Can you work these out from the model? Positions are in its coordinate system, mm. A direction names the side the tool comes from. Round coordinates to 2 decimals unless told otherwise and drop trailing zeros. Order: outer loops, then holes, each group sorted by start corner. A loop starts at its lowest first (then second) coordinate and runs counter-clockwise, first axis right, second up. Notation, with made-up numbers: (61, 36) - (109, 36) arc R27 cw to (109, 64) - close; hole circle Ø1 at (18.25, -26). An arc over 180 degrees is marked (long way). Write item = value, one per line.
from build123d import *

# Parameters (mm, degrees)
F0_R          = 40
F0_R_2        = 2
F0_R_3        = 30
F1_DEPTH      = 8
F2_R          = 40
F2_R_2        = 30
F3_DEPTH      = 2
F4_R          = 5
F5_DEPTH      = 30
F5_DEPTH_BACK = 30
F6_W          = 8
F6_H          = 1


with BuildPart() as f1:
    # F0 (on Top) → F1 (new body)
    with BuildSketch(Plane.XY):
        Circle(F0_R)
        with Locations((-30.310889, -17.5)):
            Circle(F0_R_2, mode=Mode.SUBTRACT)
        with Locations((0, -35)):
            Circle(F0_R_2, mode=Mode.SUBTRACT)
        with Locations((30.310889, -17.5)):
            Circle(F0_R_2, mode=Mode.SUBTRACT)
        with Locations((-30.310889, 17.5)):
            Circle(F0_R_2, mode=Mode.SUBTRACT)
        Circle(F0_R_3, mode=Mode.SUBTRACT)
        with Locations((30.310889, 17.5)):
            Circle(F0_R_2, mode=Mode.SUBTRACT)
        with Locations((0, 35)):
            Circle(F0_R_2, mode=Mode.SUBTRACT)
    extrude(amount=F1_DEPTH)

    # F2 (on face) → F3 (join)
    with BuildSketch(Plane.XY.offset(8)):
        Circle(F2_R)
        Circle(F2_R_2, mode=Mode.SUBTRACT)
    extrude(amount=F3_DEPTH)

    # F4 (on Front) → F5 (join, two sides)
    with BuildSketch(Plane.XZ) as f5_sk:
        with Locations((0, 5)):
            Circle(F4_R)
    extrude(amount=F5_DEPTH)
    extrude(f5_sk.sketch, amount=-F5_DEPTH_BACK)

    # F6 (on Right) → F7 (revolve, cut)
    with BuildSketch(Plane.YZ):
        with Locations((11, 9.5)):
            Rectangle(F6_W, F6_H)
        with Locations((-11, 9.5)):
            Rectangle(F6_W, F6_H)
    revolve(axis=Axis((0, 0, 5), (0, -1, 0)), mode=Mode.SUBTRACT)


solid = f1.part
(1) Will these pins go through, and if not, where does the flat tip stop? P1, Ø2, axis at y = -12.5, z = 2, coming from the -X side; P2, Ø1.5, axis at y = -13, z = 7, coming from the -X side; P3, Ø1.2, axis at x = 30, y = 17.5, coming from the -Z side.
Computed:
P1 = -38.31
P2 = -38.08
P3 = 8
(2) If I drill on line 1 (Y direction, x = 0, z = 3.5); line 2 (Y direction, x = -2, z = 9.5); line 3 (Y direction, x = 17.5, z = 2.5), over which ranges is the centre line in solid material (lowest first)? Write a range as from..to.
Computed:
line_1 = -40..-37, -33..33, 37..40
line_2 = -39.95..-15, -7..7, 15..39.95
line_3 = -35.97..-24.37, 24.37..35.97
(3) If we section it at D-D (x = -3): Write out the boundary of the cut face in (y, z), plus the area to 3 significant figures.
Computed:
outline = (-39.89, 0) - (-29.85, 0) - (-29.85, 1) - (-15, 1) - (-15, 2.35) - (-7, 2.35) - (-7, 1) - (7, 1) - (7, 2.35) - (15, 2.35) - (15, 1) - (29.85, 1) - (29.85, 0) - (39.89, 0) - (39.89, 10) - (29.85, 10) - (29.85, 9) - (15, 9) - (15, 7.65) - (7, 7.65) - (7, 9) - (-7, 9) - (-7, 7.65) - (-15, 7.65) - (-15, 9) - (-29.85, 9) - (-29.85, 10) - (-39.89, 10) - close
area = 635 mm^2
(4) If we section it at B-B (x = 15): Write out the boundary of the cut face in (y, z).
Computed:
outline = (-37.08, 0) - (-25.98, 0) - (-25.98, 10) - (-37.08, 10) - close; (25.98, 0) - (37.08, 0) - (37.08, 10) - (25.98, 10) - close
(5) If we section it at C-C (y = 22): Write out the boundary of the cut face in (x, z), plus the area to 3 significant figures.
Computed:
outline = (-33.41, 0) - (-20.4, 0) - (-20.4, 10) - (-33.41, 10) - close; circle Ø10 at (0, 5); (20.4, 0) - (33.41, 0) - (33.41, 10) - (20.4, 10) - close
area = 339 mm^2
(6) If we section it at A-A (y = 0): Write out the boundary of the cut face in (x, z).
Computed:
outline = (-40, 0) - (-30, 0) - (-30, 10) - (-40, 10) - close; circle Ø10 at (0, 5); (30, 0) - (40, 0) - (40, 10) - (30, 10) - close
(7) Thinking about a two-plate mould opening in Y: for faces 1 (the face through (-6, 30, 0)), 2 (the face through (29.993, -0.66, 4.93)), 3 (the face through (-8.67, -39.05, 4.93)), which applies, +Y half, -Y half, draft (parallel to the pull), parting line (faces both ways), or undercut?
Computed:
face_1 = draft
face_2 = undercut
face_3 = parting line
(8) On a 3-axis mill with a long thin cutter (end or side, diameter ignored), from which of +Z, -Z, +X, -X, +Y, -Y can I reach the whole of each face in a straight line? I mean faces 4 (the face through (3.905, -10.944, 4.133)), 5 (the face through (30, -17, 8)). Say none if no direction works.
Computed:
face_4 = none
face_5 = -Z
